The model under review builds one solid part; all positions refer to its coordinate system, in mm. A direction names the side the tool comes from. Coordinates: 2 decimals unless noted, no trailing zeros. Loops run counter-clockwise (first coordinate to the right, second up) from the corner with the lowest first, then second, coordinate; pieces in that order, holes last. Notation, with made-up numbers: M 71,-11 L 119,-11 A28 cw 119,12 Z; hole C 11,18.5 d3. An arc over 180 degrees is marked long. Use one line per item in the form item = value.
```python
from build123d import *

# Parameters (mm, degrees)
F0_R      = 11
F1_DEPTH  = 9.5
F2_R      = 8
F3_DEPTH  = 0.5
F4_R      = 5
F5_DEPTH  = 25
F6_R      = 5
F6_R_2    = 2.5
F7_DEPTH  = 1
F8_R      = 5
F8_R_2    = 4
F9_DEPTH  = 0.5
F10_W     = 63.0000028759
F10_H     = 42.9000016302
F11_DEPTH = 25
F13_DEPTH = 9.5
F14_R     = 1.75
F15_DEPTH = 25


with BuildPart() as f1:
    # F0 (on Top) → F1 (new body)
    with BuildSketch(Plane.XY):
        Circle(F0_R)
    extrude(amount=F1_DEPTH)

    # F2 (on face) → F3 (cut)
    with BuildSketch(Plane.XY.offset(9.5)):
        Circle(F2_R)
    extrude(amount=-F3_DEPTH, mode=Mode.SUBTRACT)

    # F4 (on face) → F5 (cut)
    with BuildSketch(Plane.XY.offset(9)):
        Circle(F4_R)
    extrude(amount=-F5_DEPTH, mode=Mode.SUBTRACT)

    # F6 (on face) → F7 (join)
    with BuildSketch(Plane(origin=(0, 0, 0), x_dir=(1, 0, 0), z_dir=(0, 0, -1))):
        Circle(F6_R)
        Circle(F6_R_2, mode=Mode.SUBTRACT)
    extrude(amount=-F7_DEPTH)

    # F8 (on face) → F9 (join)
    with BuildSketch(Plane.XY.offset(1)):
        Circle(F8_R)
        Circle(F8_R_2, mode=Mode.SUBTRACT)
    extrude(amount=F9_DEPTH)

    # F10 (on Right) → F11 (cut)
    with BuildSketch(Plane.YZ):
        with Locations((3.45000159, 3.6000004038)):
            Rectangle(F10_W, F10_H)
    extrude(amount=-F11_DEPTH, mode=Mode.SUBTRACT)

    # F12 (on Top) → F13 (join)
    with BuildSketch(Plane.XY):
        with BuildLine():
            ThreePointArc((4, -10.246950766), (2.0351340956, -10.810098483), (0, -11))
            Line((0, -11), (0, -19))
            Line((0, -19), (4, -19))
            Line((4, -19), (4, -10.246950766))
        make_face()
        with BuildLine():
            Line((0, 19), (0, 11))
            ThreePointArc((0, 11), (2.0351340956, 10.810098483), (4, 10.246950766))
            Line((4, 10.246950766), (4, 19))
            Line((4, 19), (0, 19))
        make_face()
    extrude(amount=F13_DEPTH)

    # F14 (on face) → F15 (cut)
    with BuildSketch(Plane.YZ.offset(4)):
        with Locations((-15, 4.75)):
            Circle(F14_R)
        with Locations((15, 4.75)):
            Circle(F14_R)
    extrude(amount=-F15_DEPTH, mode=Mode.SUBTRACT)


solid = f1.part
```
1. Add section D-D (y = 0). State the section outline as (x, z) points, then the cut area to 3 significant figures.
Response values:
outline = M 2.5,0 L 11,0 L 11,9.5 L 8,9.5 L 8,9 L 5,9 L 5,1.5 L 4,1.5 L 4,1 L 2.5,1 Z
area = 58.5 mm^2
2. Add section C-C (x = 1.5). State the section outline as (y, z) points.
Response values:
outline = M -19,0 L -2,0 L -2,1 L -3.71,1 L -3.71,1.5 L -4.77,1.5 L -4.77,9 L -7.86,9 L -7.86,9.5 L -19,9.5 Z; M 2,0 L 19,0 L 19,9.5 L 7.86,9.5 L 7.86,9 L 4.77,9 L 4.77,1.5 L 3.71,1.5 L 3.71,1 L 2,1 Z; hole C -15,4.75 d3.5; hole C 15,4.75 d3.5
3. Add section B-B (y = 15). State the section outline as (x, z) points, then the cut area to 3 significant figures.
Response values:
outline = M 0,0 L 4,0 L 4,3 L 0,3 Z; M 0,6.5 L 4,6.5 L 4,9.5 L 0,9.5 Z
area = 24.0 mm^2
4. Add section A-A (z = 4.75). State the section outline as (x, y) points, then the cut area to 3 significant figures.
Response values:
outline = M 0,-19 L 4,-19 L 4,-16.75 L 0,-16.75 Z; M 0,-13.25 L 4,-13.25 L 4,-10.25 A11 ccw 4,10.25 L 4,13.25 L 0,13.25 L 0,5 A5 cw 0,-5 Z; M 0,16.75 L 4,16.75 L 4,19 L 0,19 Z
area = 189 mm^2
5. Insertion check: P1, Ø4.5, axis at y = -15, z = 4.75, coming from the +X side; P2, Ø2, axis at x = 9, z = 2.5, coming from the -Y side; P3, Ø1.2, axis at x = 2.5, y = -2, coming from the +Z side. Each pin has a flat end and moves straight along its axis. Give the tip position at first contact, or say it passes through.
Response values:
P1 = 4
P2 = -7.55
P3 = 1
6. Machinability: for faces 4 (the face through (6, 0, 9)), 5 (the face through (4, -13, 5)), 6 (the face through (4, 0, 0)), which of the approach directions +Z, -Z, +X, -X, +Y, -Y give a long, thin tool a straight path to every point of the face, cutting with its end or side? Answer none if there is none.
Response values:
face_4 = +Z, -X
face_5 = +Z, -Z, +X, -Y
face_6 = -Z, +X, -X, +Y, -Y
7. The part is to be moulded in two halves that separate along Z. For faces 1 (the face through (4.2, 0, 1.5)), 2 (the face through (2.03, 15.81, 3.2)), 3 (the face through (4, 13, 5)), say which applies: pulls with the +Z half, pulls with the -Z half, needs draft (parallel to the pull), parting line crosses it, or undercut.
Response values:
face_1 = pulls with the +Z half
face_2 = undercut
face_3 = needs draft
8. Wall thickness on line 1 along Z through (x, y) = (1, -15); line 2 along Y through (x, z) = (1.75, 6.25); line 3 along X through (y, z) = (11, 8.25): over which ranges is each line inside the solid? List them lowest first. Write a range as from..to.
Response values:
line_1 = 0..3, 6.5..9.5
line_2 = -19..-15.9, -14.1..-4.68, 4.68..14.1, 15.9..19
line_3 = 0..4
